Check sheet for the drawn part. Datum: minimum x, y, z corner. Units: mm. A direction names the side the tool comes from. Give positions to 0.01 mm unless a question says otherwise; leave off trailing zeros. Write each loop counter-clockwise with the first axis right and the second up, starting at its lowest first coordinate (ties: lowest second). Pieces come first, ordered by that corner, then holes. Notation, with made-up numbers: (48, -30) - (81, -30) arc R3 ccw to (81, -25) - close; hole circle Ø8 at (-4, 7.25). An arc over 180 degrees is marked (long way). One line per question, with ' | ' between items. Start each with the question number.
Q1. Section check B-B on z = 70. Record the boundary of the cut face in (x, y).
Q2. Section check D-D on z = 21.75. Record the boundary of the cut face in (x, y).
Q3. Set-up check for the marked faces 1, 2 and 3: record each of +Z, -Z, +X, -X, +Y, -Y from which the full face is reachable in a straight line by a thin tool's end or side.
Q4. Gauge pin test, flat ends, axial feed: P1, Ø4.5, axis at x = 81.75, z = 28.25, coming from the +Y side; P2, Ø3, axis at x = 6, y = 4.5, coming from the +Z side; P3, Ø8, axis at x = 79.5, y = 17, coming from the -Z side. Record the tip position at first contact, or that the pin passes through.
Q5. Section check C-C on y = 12.5. Record the boundary of the cut face in (x, z).
Q6. Thickness scan on L1, parallel to Z at x = 10, y = 15.5; L2, parallel to X at y = 12.75, z = 70; L3, parallel to Z at x = 10, y = 8. Record the ranges inside material, lowest first. Write a range as [from, to].
Q7. Section check A-A on x = 85. Record the boundary of the cut face in (y, z), and give its area (3 significant figures).
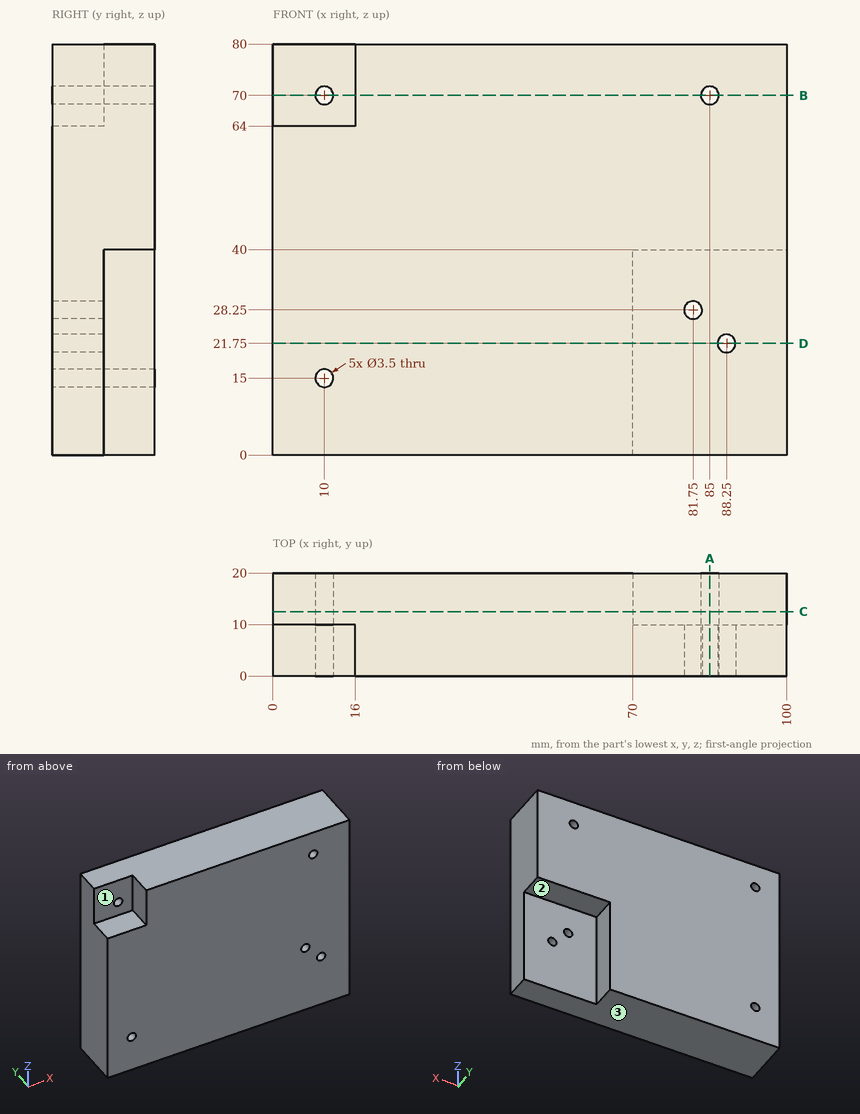
Working result:
1) outline: (0, 10) - (8.25, 10) - (8.25, 20) - (0, 20) - close; (11.75, 10) - (16, 10) - (16, 0) - (83.25, 0) - (83.25, 20) - (11.75, 20) - close; (86.75, 0) - (100, 0) - (100, 20) - (86.75, 20) - close
2) outline: (0, 0) - (86.5, 0) - (86.5, 10) - (70, 10) - (70, 20) - (0, 20) - close; (90, 0) - (100, 0) - (100, 10) - (90, 10) - close
3) face 1: +Z, -X, -Y | face 2: -Z, +X, +Y | face 3: -Z, +X, -X, +Y, -Y
4) P1: stops at y = 10 | P2: stops at z = 64 | P3: stops at z = 40
5) outline: (0, 0) - (70, 0) - (70, 40) - (100, 40) - (100, 80) - (0, 80) - close; hole circle Ø3.5 at (10, 15); hole circle Ø3.5 at (10, 70); hole circle Ø3.5 at (85, 70)
6) L1: z = [0, 13.25], [16.75, 68.25], [71.75, 80] | L2: x = [0, 8.25], [11.75, 83.25], [86.75, 100] | L3: z = [0, 13.25], [16.75, 64]
7) outline: (0, 0) - (10, 0) - (10, 40) - (20, 40) - (20, 68.25) - (0, 68.25) - close; (0, 71.75) - (20, 71.75) - (20, 80) - (0, 80) - close | area: 1,130 mm2
